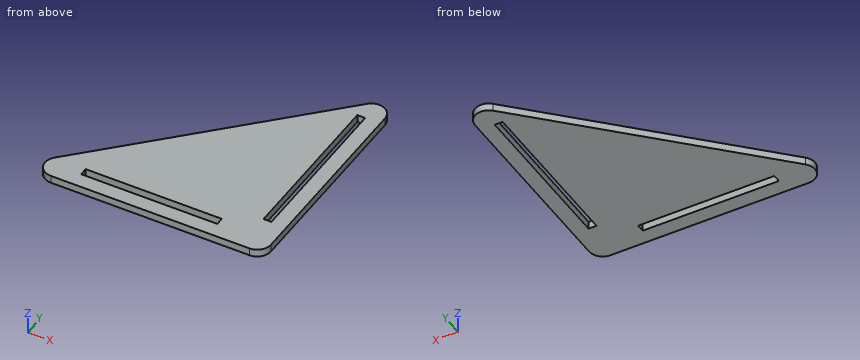
```python
from build123d import *

# Parameters (mm, degrees)
SKETCH_1_W      = 2.9
SKETCH_1_H      = 60
SKETCH_1_W_2    = 50
SKETCH_1_H_2    = 2.9
EXTRUDE_1_DEPTH = 1.4


with BuildPart() as part:
    # Эскиз1 → Бобышка-Вытянуть1 (new, symmetric)
    with BuildSketch(Plane.XY):
        with BuildLine():
            Line((-36.464466094, -36.464466094), (36.464466094, 36.464466094))
            ThreePointArc((36.464466094, 36.464466094), (41.913417162, 37.548329851), (45, 32.928932188))
            Line((45, 32.928932188), (45, -40))
            ThreePointArc((45, -40), (43.535533906, -43.535533906), (40, -45))
            Line((40, -45), (-32.928932188, -45))
            ThreePointArc((-32.928932188, -45), (-37.548329851, -41.913417162), (-36.464466094, -36.464466094))
        make_face()
        with Locations((38, 0)):
            Rectangle(SKETCH_1_W, SKETCH_1_H, mode=Mode.SUBTRACT)
        with Locations((0, -38)):
            Rectangle(SKETCH_1_W_2, SKETCH_1_H_2, mode=Mode.SUBTRACT)
    extrude(amount=EXTRUDE_1_DEPTH, both=True)


solid = part.part
```
Geometry: final body of the model. Coordinates: model frame, mm. Coordinates: 2 decimals unless noted, no trailing zeros. Order: outer loops, then holes, each group sorted by start corner. A loop starts at its lowest first (then second) coordinate and runs counter-clockwise, first axis right, second up. Notation, with made-up numbers: M -25.75,-36.75 L -3.75,-36.75 A17 ccw -3.75,-28.75 Z; hole C 29,23 d6. An arc over 180 degrees is marked long. Answer in a Markdown table with one row per item. Add a question column.
Q1. Section query A-A on y = -8.5. Return the cut outline in (x, z).
Q2. Section query C-C on z = -0.8. Return the cut outline in (x, y), and give its area (3 significant figures).
Q3. Section query B-B on x = -19. Return the cut outline in (y, z).
Q4. Section query D-D on x = -30. Return the cut outline in (y, z).
Q5. Contact query for flat-ended pins moving along their axis: P1, Ø1, axis at x = -20, z = -0.5, coming from the +Y side; P2, Ø1.4, axis at x = -3.5, z = 0, coming from the +Y side. Output: stop coordinate, or through.
Q6. Line query: L1, parallel to X at y = 5, z = -0.85; L2, parallel to Y at x = -10.5, z = -1.2; L3, parallel to Y at x = 20.5, z = -0.25. Output: solid intervals per line, ascending.
Completed:
| question | item | result |
|---|---|---|
| 1 | outline | M -8.5,-1.4 L 36.55,-1.4 L 36.55,1.4 L -8.5,1.4 Z; M 39.45,-1.4 L 45,-1.4 L 45,1.4 L 39.45,1.4 Z |
| 2 | outline | M -36.46,-36.46 A5 ccw -32.93,-45 L 40,-45 A5 ccw 45,-40 L 45,32.93 A5 ccw 36.46,36.46 Z; hole M -25,-39.45 L 25,-39.45 L 25,-36.55 L -25,-36.55 Z; hole M 36.55,-30 L 39.45,-30 L 39.45,30 L 36.55,30 Z |
| 2 | area | 3,660 mm2 |
| 3 | outline | M -45,-1.4 L -39.45,-1.4 L -39.45,1.4 L -45,1.4 Z; M -36.55,-1.4 L -19,-1.4 L -19,1.4 L -36.55,1.4 Z |
| 4 | outline | M -45,-1.4 L -30,-1.4 L -30,1.4 L -45,1.4 Z |
| 5 | P1 | stops at y = -19.5 |
| 5 | P2 | stops at y = -2.8 |
| 6 | L1 | x = 5 to 36.55, 39.45 to 45 |
| 6 | L2 | y = -45 to -39.45, -36.55 to -10.5 |
| 6 | L3 | y = -45 to -39.45, -36.55 to 20.5 |
